Autodesk Inventor part; units mm, degrees
ref_plane "YZ Plane" through (0, 0, 0) normal (1, 0, 0) x (0, 1, 0)
ref_plane "XZ Plane" through (0, 0, 0) normal (0, 1, 0) x (-1, 0, 0)
ref_plane "XY Plane" through (0, 0, 0) normal (0, 0, 1) x (1, 0, 0)
sketch "草图1" plane through (0, 0, 0) normal (0, 1, 0) x (-1, 0, 0)
  line L0 (0, 0) -> (-90, 0)
  line L1 (-90, 0) -> (-90, -140)
  line L2 (-90, -140) -> (0, -140)
  line L3 (0, -140) -> (0, 0)
  point P0 (-45, -70)
  dimension "d0" = 140
  dimension "d1" = 90
extrude "拉伸1" add sketch "草图1" along normal blind 25
sketch "草图2" plane through (0, 25, 0) normal (0, 1, 0) x (1, 0, 0)
  line L0 (90, 0) -> (90, 140)
  line L1 (90, 140) -> (0, 140)
  line L2 (0, 140) -> (0, 0)
  line L3 (0, 0) -> (90, 0)
  line L4 (5, 5) -> (85, 5)
  line L5 (85, 5) -> (85, 135)
  line L6 (85, 135) -> (5, 135)
  line L7 (5, 135) -> (5, 5)
  line L8 (5, 5) -> (85, 135) construction
  line L9 (85, 5) -> (5, 135) construction
  point P0 (45, 70)
  dimension "d4" = 80
  dimension "d5" = 130
extrude "拉伸2" cut sketch "草图2" against normal blind 23.8 contours L7 L6 L5 L4
fillet "面圆角1" radius 5 1 edges at (5, 13.1, -5)
fillet "面圆角2" radius 5 1 edges at (5, 13.1, -135)
fillet "面圆角3" radius 5 1 edges at (85, 13.1, -135)
fillet "面圆角4" radius 5 1 edges at (85, 13.1, -5)
sketch "草图4" plane through (0, 1.2, 0) normal (0, 1, 0) x (1, 0, 0)
  arc A0 (80, 5) -> (85, 10) centre (80, 10) ccw
  line L0 (85, 130) -> (85, 10)
  arc A1 (85, 130) -> (80, 135) centre (80, 130) ccw
  line L1 (10, 135) -> (80, 135)
  arc A2 (10, 135) -> (5, 130) centre (10, 130) ccw
  line L2 (5, 10) -> (5, 130)
  arc A3 (5, 10) -> (10, 5) centre (10, 10) ccw
  line L3 (80, 5) -> (10, 5)
  line L4 (16.152, 18.12) -> (14.152, 18.12)
  line L5 (11.152, 15.12) -> (11.152, 13.12)
  line L6 (14.152, 10.12) -> (16.152, 10.12)
  line L7 (19.152, 13.12) -> (19.152, 15.12)
  line L8 (19.152, 18.12) -> (11.152, 10.12) construction
  line L9 (11.152, 18.12) -> (19.152, 10.12) construction
  arc A4 (11.152, 13.12) -> (14.152, 10.12) centre (14.152, 13.12) ccw
  arc A5 (16.152, 10.12) -> (19.152, 13.12) centre (16.152, 13.12) ccw
  arc A6 (19.152, 15.12) -> (16.152, 18.12) centre (16.152, 15.12) ccw
  arc A7 (14.152, 18.12) -> (11.152, 15.12) centre (14.152, 15.12) ccw
  line L10 (15.152, 14.12) -> (74.848, 14.12)
  line L11 (15.152, 14.12) -> (15.152, 125.88)
  line L12 (70.848, 15.12) -> (70.848, 13.12)
  arc A8 (70.848, 13.12) -> (73.848, 10.12) centre (73.848, 13.12) ccw
  line L13 (73.848, 10.12) -> (75.848, 10.12)
  arc A9 (75.848, 10.12) -> (78.848, 13.12) centre (75.848, 13.12) ccw
  line L14 (78.848, 13.12) -> (78.848, 15.12)
  arc A10 (78.848, 15.12) -> (75.848, 18.12) centre (75.848, 15.12) ccw
  line L15 (75.848, 18.12) -> (73.848, 18.12)
  arc A11 (73.848, 18.12) -> (70.848, 15.12) centre (73.848, 15.12) ccw
  line L16 (11.152, 126.88) -> (11.152, 124.88)
  arc A12 (11.152, 124.88) -> (14.152, 121.88) centre (14.152, 124.88) ccw
  line L17 (14.152, 121.88) -> (16.152, 121.88)
  arc A13 (16.152, 121.88) -> (19.152, 124.88) centre (16.152, 124.88) ccw
  line L18 (19.152, 124.88) -> (19.152, 126.88)
  arc A14 (19.152, 126.88) -> (16.152, 129.88) centre (16.152, 126.88) ccw
  line L19 (16.152, 129.88) -> (14.152, 129.88)
  arc A15 (14.152, 129.88) -> (11.152, 126.88) centre (14.152, 126.88) ccw
  line L20 (70.848, 126.88) -> (70.848, 124.88)
  arc A16 (70.848, 124.88) -> (73.848, 121.88) centre (73.848, 124.88) ccw
  line L21 (73.848, 121.88) -> (75.848, 121.88)
  arc A17 (75.848, 121.88) -> (78.848, 124.88) centre (75.848, 124.88) ccw
  line L22 (78.848, 124.88) -> (78.848, 126.88)
  arc A18 (78.848, 126.88) -> (75.848, 129.88) centre (75.848, 126.88) ccw
  line L23 (75.848, 129.88) -> (73.848, 129.88)
  arc A19 (73.848, 129.88) -> (70.848, 126.88) centre (73.848, 126.88) ccw
  point P0 (0, 0)
  point P1 (45, 70)
  point P2 (45, 70)
  point P3 (70.848, 10.12)
  point P4 (70.848, 18.12)
  point P5 (78.848, 10.12)
  point P6 (78.848, 18.12)
  point P7 (11.152, 121.88)
  point P8 (11.152, 129.88)
  point P9 (19.152, 121.88)
  point P10 (19.152, 129.88)
  point P11 (70.848, 121.88)
  point P12 (70.848, 129.88)
  point P13 (78.848, 121.88)
  point P14 (78.848, 129.88)
  dimension "d12" = 55.88
  dimension "d13" = 29.848
  dimension "d14" = 8
  dimension "d15" = 8
  dimension "d16" = 3
  dimension "d17" = 59.696
  dimension "d18" = 111.76
  dimension "d21" = 59.696
  dimension "d24" = 111.76
extrude "拉伸3" add sketch "草图4" along normal blind 8 contours A6 L7 L10 L11 L4 | L11 L10 L7 A5 L6 A4 L5 A7 L4 | A11 L15 A10 L14 A9 L13 A8 L12 | A15 L19 A14 L18 A13 L17 A12 L16 | A19 L23 A18 L22 A17 L21 A16 L20
properties part number "PrismGC"
Model file for the job. Use its own axes, mm. A direction names the side the tool comes from. Give positions to 0.01 mm unless a question says otherwise; leave off trailing zeros. Order: outer loops, then holes, each group sorted by start corner. A loop starts at its lowest first (then second) coordinate and runs counter-clockwise, first axis right, second up. Notation, with made-up numbers: M 63,27 L 75,27 A15 cw 75,42 Z; hole C 66,72 d3. An arc over 180 degrees is marked long. Write item = value, one per line.
Q1. Cut at D-D, the plane x = 30. List the corners of the cut face in (y, z).
Derived:
outline = M 0,-140 L 25,-140 L 25,-135 L 1.2,-135 L 1.2,-5 L 25,-5 L 25,0 L 0,0 Z
Q2. Two-plate mould, pull along Z, no slides. Class faces 1 (the flat face through (46, 12, -140)), 2 (the cylindrical face through (83, 13, -134)), 3 (the flat face through (90, 12, -69)), 4 (the cylindrical face through (12.01, 5.14, -17.22)): pulls with the +Z half, pulls with the -Z half, needs draft (parallel to the pull), parting line crosses it, or undercut.
Derived:
face_1 = pulls with the -Z half
face_2 = undercut
face_3 = needs draft
face_4 = undercut
Q3. Drill centre lines: line 1 (Z direction, x = 64, y = 8); line 2 (X direction, y = 8, z = -62.5); line 3 (Z direction, x = 72, y = 4.5). Where is each one in solid material? Low to high. Write a range as [from, to].
Derived:
line_1 = [-140, -135], [-5, 0]
line_2 = [0, 5], [85, 90]
line_3 = [-140, -135], [-129.24, -122.52], [-17.48, -10.76], [-5, 0]
Q4. Cut at C-C, the plane y = 5. Count the separate pieces of the cut face and the enclosed holes in it, then the cut area to 3 significant figures.
Derived:
separate_pieces = 5
enclosed_holes = 1
area = 2,450 mm2
Q5. Tool access for faces 5 (the cylindrical face through (12.05, 5.14, -10.98)), 6 (the flat face through (44, 12, 0)): list every direction of +Z, -Z, +X, -X, +Y, -Y with a clear straight run to the whole face (end or side of a thin tool).
Derived:
face_5 = +Y
face_6 = +Z, +X, -X, +Y, -Y
Q6. Cut at B-B, the plane z = -53.5. List the corners of the cut face in (x, y), then the cut area to 3 significant figures.
Derived:
outline = M 0,0 L 90,0 L 90,25 L 85,25 L 85,1.2 L 5,1.2 L 5,25 L 0,25 Z
area = 346 mm2
Q7. Flat gauge pins, fed straight in: pin 1 (4 mm diameter, centred on x = 15.5, z = -127.5, fed in from +Y); pin 2 (8 mm diameter, centred on x = 33.5, z = -67, fed in from +Y). Where does each tip first touch, or does it go through?
Derived:
pin_1 = 9.2
pin_2 = 1.2
Q8. Cut at A-A, the plane y = 21.75. List the corners of the cut face in (x, z), then the cut area to 3 significant figures.
Derived:
outline = M 0,-140 L 90,-140 L 90,0 L 0,0 Z; hole M 5,-130 A5 ccw 10,-135 L 80,-135 A5 ccw 85,-130 L 85,-10 A5 ccw 80,-5 L 10,-5 A5 ccw 5,-10 Z
area = 2,220 mm2
